Input: part model. Units: mm. Frame: model coordinates. Round coordinates to 2 decimals unless told otherwise and drop trailing zeros. Loops run counter-clockwise (first coordinate to the right, second up) from the corner with the lowest first, then second, coordinate; pieces in that order, holes last.
(1) Cut plane A-A, the plane z = 6. Output: boundary loops of the cut face in (x, y).
(2) Cut plane B-B, the plane x = 37.5. Output: boundary loops of the cut face in (y, z).
(3) First-contact query: pin 1 Ø2 at (y, z) = (9.5, 4.5) entering from -X; pin 2 Ø1 at (y, z) = (-6.5, 4.5) entering from +X; pin 3 Ø2 at (x, y) = (-5, 10) entering from -Z; pin 4 Ø3.5 at (x, z) = (30.5, 5.5) entering from +Y. Flat tips, straight axial feed; report the tip coordinate or a pass-through.
(4) Cut plane C-C, the plane y = 3. Give the number of separate pieces and of enclosed holes in the cut face, and give its area (3 significant figures).
(5) Line query: line 1 (X direction, y = 2.25, z = 7); line 2 (X direction, y = -5, z = 2.5); line 3 (X direction, y = -7.25, z = 6.75). Output: solid intervals per line, ascending.
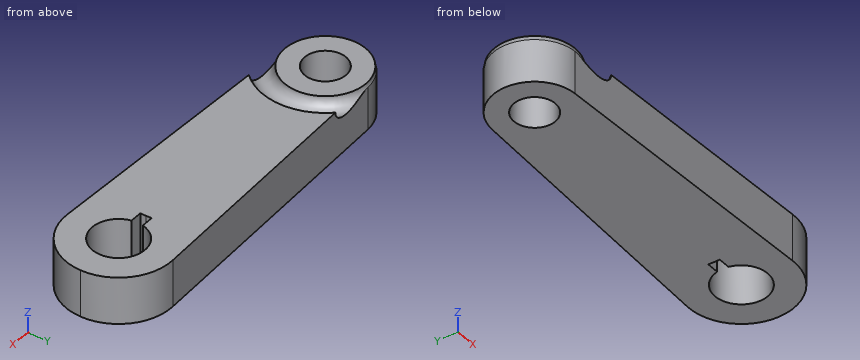
from build123d import *

# Parameters (mm, degrees)
F0_R     = 5.5
F1_DEPTH = 12.5
F2_R     = 3


with BuildPart() as f1:
    # F0 (on Top) → F1 (new body)
    with BuildSketch(Plane.XY):
        with BuildLine():
            ThreePointArc((-37.176539, -10.991427), (-29.119216, -7.930205), (-25.742329, 0))
            ThreePointArc((-25.742329, 0), (-29.119216, 7.930205), (-37.176539, 10.991427))
            ThreePointArc((-37.176539, 10.991427), (-47.742329, 0), (-37.176539, -10.991427))
        make_face()
        with Locations((-36.742329, 0)):
            Circle(F0_R, mode=Mode.SUBTRACT)
        with BuildLine():
            ThreePointArc((53.257671, 0), (48.959814, 10.092989), (38.70504, 13.989089))
            ThreePointArc((38.70504, 13.989089), (25.257671, 0), (38.70504, -13.989089))
            ThreePointArc((38.70504, -13.989089), (48.959814, -10.092989), (53.257671, 0))
        make_face()
        with BuildLine():
            ThreePointArc((32.420274, 1.5), (46.257671, 0), (32.420274, -1.5))
            Line((32.420274, -1.5), (29.227967, -1.5))
            Line((29.227967, -1.5), (29.227967, 0))
            Line((29.227967, 0), (29.168711, 1.5))
            Line((29.168711, 1.5), (32.420274, 1.5))
        make_face(mode=Mode.SUBTRACT)
        with BuildLine():
            ThreePointArc((-37.176539, 10.991427), (-29.119216, 7.930205), (-25.742329, 0))
            ThreePointArc((-25.742329, 0), (-29.119216, -7.930205), (-37.176539, -10.991427))
            Line((-37.176539, -10.991427), (38.70504, -13.989089))
            ThreePointArc((38.70504, -13.989089), (25.257671, 0), (38.70504, 13.989089))
            Line((38.70504, 13.989089), (-37.176539, 10.991427))
        make_face()
    extrude(amount=F1_DEPTH)

    # F2 (on Front) → F3 (revolve, cut)
    with BuildSketch(Plane.XZ):
        with Locations((-50.519399, 12.484903)):
            Circle(F2_R)
    revolve(axis=Axis((-36.742329, 0, 0), (0, 0, -1)), mode=Mode.SUBTRACT)


solid = f1.part
Reported:
1. outline: (-37.18, -10.99) - (38.71, -13.99) arc R14 ccw (long way) to (38.71, 13.99) - (-37.18, 10.99) arc R11 ccw to start; hole circle Ø11 at (-36.74, 0); hole (29.17, 1.5) - (29.23, 0) - (29.23, -1.5) - (32.42, -1.5) arc R7 ccw (long way) to (32.42, 1.5) - close
2. outline: (-13.94, 0) - (-6.78, 0) - (-6.78, 12.5) - (-13.94, 12.5) - close; (6.78, 0) - (13.94, 0) - (13.94, 12.5) - (6.78, 12.5) - close
3. pin 1: stops at x = -43.72
3. pin 2: stops at x = 51.91
3. pin 3: stops at z = 0
3. pin 4: stops at y = 13.73
4. separate pieces: 3
4. enclosed holes: 0
4. area: 965 mm2
5. line 1: x = -47.51 to -41.76, -31.72 to 32.63, 45.89 to 53.08
5. line 2: x = -46.54 to -39.03, -34.45 to 34.36, 44.16 to 52.33
5. line 3: x = -45.02 to 51.23
